The model under review builds one solid part; all positions refer to its coordinate system, in mm. Face numbers are marked on the shaded views. A direction names the side the tool comes from. Round coordinates to 2 decimals unless told otherwise and drop trailing zeros. Write each loop counter-clockwise with the first axis right and the second up, starting at its lowest first coordinate (ties: lowest second). Pieces come first, ordered by that corner, then holes. Notation, with made-up numbers: (51.25, -15.5) -> (82.25, -15.5) arc R33 ccw to (82.25, 22.5) -> close; hole circle Ø11 at (8.25, 75.5). An arc over 180 degrees is marked (long way). Return JSON: item names as keys, results as strings. Group by question number.
1. Take a section at C-C, the plane z = 12.5. Write out the cut boundary in (x, y), then the cut area to 3 significant figures.
2. Take a section at B-B, the plane y = 2. Write out the cut boundary in (x, z), then the cut area to 3 significant figures.
3. Take a section at D-D, the plane x = 17.5. Write out the cut boundary in (y, z), then the cut area to 3 significant figures.
4. Tool access review of the marked faces 1 and 2: name each direction out of +Z, -Z, +X, -X, +Y, -Y from which nothing blocks a thin tool from reaching the whole face with its end or side.
5. Take a section at A-A, the plane z = 34. Write out the cut boundary in (x, y).
6. Mouldability with a two-part tool opening along X and no side actions: class the marked faces 3, 4, 5 and 6 as pulls with the +X half, pulls with the -X half, needs draft (parallel to the pull), parting line crosses it, or undercut.
7. For line 1 along X through (y, z) = (-2.25, 17.5); line 2 along Z through (x, y) = (3, 6.5); line 3 along X through (y, z) = (2.75, 33), list the stretches that pass through material, from the lowest coordinate up. Write a range as from..to.
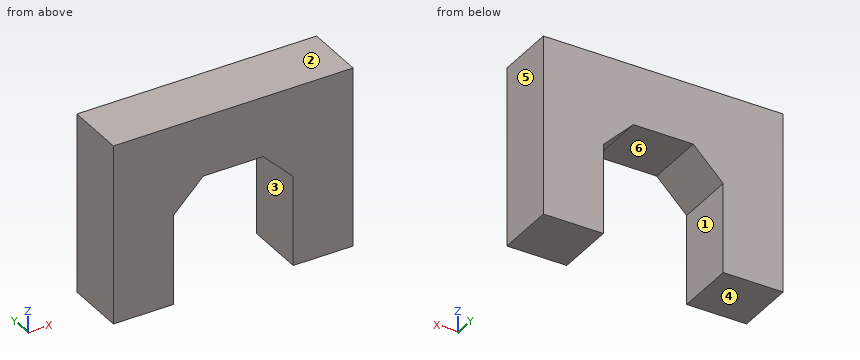
from build123d import *

# Parameters (mm, degrees)
PAD_DEPTH    = 10
CHAMFER_SIZE = 10


with BuildPart() as part:
    # Sketch → Pad (new body, symmetric)
    with BuildSketch(Plane.XZ):
        Polygon((-40, 0), (-20, 0), (-20, 40), (20, 40), (20, 0), (40, 0), (40, 60), (-40, 60), align=None)
    extrude(amount=PAD_DEPTH, both=True)

    # Chamfer
    chamfer_edges = [part.edges().sort_by_distance(p)[0] for p in [
        (-20, 0, 40),
        (20, 0, 40),
    ]]
    chamfer(chamfer_edges, length=CHAMFER_SIZE)


solid = part.part
Output:
{
 "1": {"outline": "(-40, -10) -> (-20, -10) -> (-20, 10) -> (-40, 10) -> close; (20, -10) -> (40, -10) -> (40, 10) -> (20, 10) -> close", "area": "800 mm^2"},
 "2": {"outline": "(-40, 0) -> (-20, 0) -> (-20, 30) -> (-10, 40) -> (10, 40) -> (20, 30) -> (20, 0) -> (40, 0) -> (40, 60) -> (-40, 60) -> close", "area": "3,300 mm^2"},
 "3": {"outline": "(-10, 32.5) -> (10, 32.5) -> (10, 60) -> (-10, 60) -> close", "area": "550 mm^2"},
 "4": {"face 1": "-Z, +Y, -Y", "face 2": "+Z, +X, -X, +Y, -Y"},
 "5": {"outline": "(-40, -10) -> (-16, -10) -> (-16, 10) -> (-40, 10) -> close; (16, -10) -> (40, -10) -> (40, 10) -> (16, 10) -> close"},
 "6": {"face 3": "undercut", "face 4": "needs draft", "face 5": "pulls with the +X half", "face 6": "undercut"},
 "7": {"line 1": "x = -40..-20, 20..40", "line 2": "z = 40..60", "line 3": "x = -40..-17, 17..40"}
}
